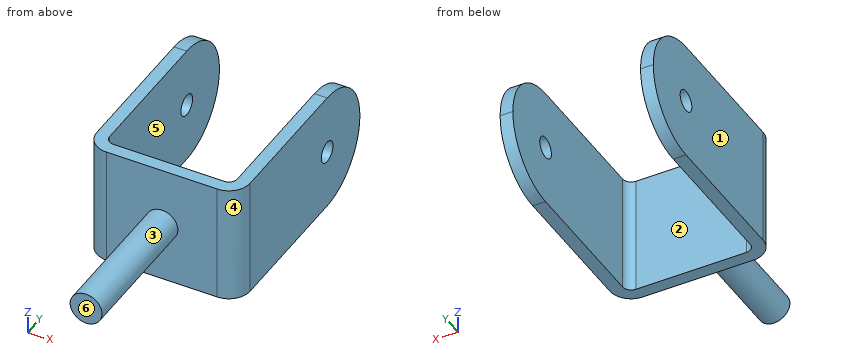
```python
from build123d import *

# Parameters (mm, degrees)
BOSS_EXTRUDE1_DEPTH     = 280
SKETCH2_R               = 25
CUT_EXTRUDE3_DEPTH      = 1
CUT_EXTRUDE3_DEPTH_BACK = 399
SKETCH4_R               = 37.5
BOSS_EXTRUDE2_DEPTH     = 325


with BuildPart() as part:
    # Sketch1 → Boss-Extrude1 (new body)
    with BuildSketch(Plane.XY):
        with BuildLine():
            Line((-130, 0), (130, 0))
            ThreePointArc((130, 0), (165.355339059, 14.644660941), (180, 50))
            Line((180, 50), (180, 520))
            Line((180, 520), (150, 520))
            Line((150, 520), (150, 50))
            ThreePointArc((150, 50), (144.142135624, 35.857864376), (130, 30))
            Line((130, 30), (-130, 30))
            ThreePointArc((-130, 30), (-144.142135624, 35.857864376), (-150, 50))
            Line((-150, 50), (-150, 520))
            Line((-150, 520), (-180, 520))
            Line((-180, 520), (-180, 50))
            ThreePointArc((-180, 50), (-165.355339059, 14.644660941), (-130, 0))
        make_face()
    extrude(amount=BOSS_EXTRUDE1_DEPTH)

    # Sketch2 → Cut-Extrude3 (cut, two sides)
    with BuildSketch(Plane.ZY.offset(180)) as cut_extrude3_sk:
        with BuildLine():
            Line((280, 520), (140, 520))
            ThreePointArc((140, 520), (238.994949366, 478.994949366), (280, 380))
            Line((280, 380), (280, 520))
        make_face()
        with BuildLine():
            Line((0, 520), (0, 380))
            ThreePointArc((0, 380), (41.005050634, 478.994949366), (140, 520))
            Line((140, 520), (0, 520))
        make_face()
        with Locations((140, 380)):
            Circle(SKETCH2_R)
    extrude(amount=CUT_EXTRUDE3_DEPTH, mode=Mode.SUBTRACT)
    extrude(cut_extrude3_sk.sketch, amount=-CUT_EXTRUDE3_DEPTH_BACK, mode=Mode.SUBTRACT)

    # Sketch4 → Boss-Extrude2 (add)
    with BuildSketch(Plane.XZ):
        with Locations((0, 140)):
            Circle(SKETCH4_R)
    extrude(amount=BOSS_EXTRUDE2_DEPTH)


solid = part.part
```
Geometry check sheet. Reference: the model listing, model coordinates, mm. Face numbers are marked on the shaded views. A direction names the side the tool comes from. Give positions to 0.01 mm unless a question says otherwise; leave off trailing zeros. Order: outer loops, then holes, each group sorted by start corner. A loop starts at its lowest first (then second) coordinate and runs counter-clockwise, first axis right, second up.
1. Section check C-C, the plane z = 221. Enter the section's corners in (x, y).
2. Section check B-B, the plane x = 0. Enter the section's corners in (y, z).
3. Access from +Z, -Z, +X, -X, +Y, -Y to the whole of each face (thin tool, end or side, straight path). Record for the marked faces 1, 2 and 3.
4. Thickness scan on L1, parallel to X at y = 440.5, z = 234; L2, parallel to Y at x = -81.5, z = 242.5; L3, parallel to Y at x = 168, z = 140. Record the ranges inside material, lowest first.
5. Section check D-D, the plane y = 452. Enter the section's corners in (x, z).
6. Release check for a two-part mould opening along X. For the marked faces 4, 5 and 6 record: pulls with the +X half, pulls with the -X half, needs draft (parallel to the pull), parting line crosses it, or undercut.
7. Gauge pin test, flat end, axial feed: pin 1 Ø2 at (y, z) = (-116, 124) entering from +X. Record the tip position at first contact, or that the pin passes through.
8. Section check A-A, the plane y = 310.5. Enter the section's corners in (x, z), and give its area (3 significant figures).
Values follow:
1. outline: (-180, 50) arc R50 ccw to (-130, 0) - (130, 0) arc R50 ccw to (180, 50) - (180, 494.19) - (150, 494.19) - (150, 50) arc R20 cw to (130, 30) - (-130, 30) arc R20 cw to (-150, 50) - (-150, 494.19) - (-180, 494.19) - close
2. outline: (-325, 102.5) - (0, 102.5) - (0, 0) - (30, 0) - (30, 280) - (0, 280) - (0, 177.5) - (-325, 177.5) - close
3. face 1: +Z, -Z, -X, +Y, -Y
3. face 2: +Z, -Z, +Y
3. face 3: -Y
4. L1: x = -180 to -150, 150 to 180
4. L2: y = 0 to 30
4. L3: y = 17.5 to 355, 405 to 520
5. outline: (-180, 19.93) - (-150, 19.93) - (-150, 260.07) - (-180, 260.07) - close; (150, 19.93) - (180, 19.93) - (180, 260.07) - (150, 260.07) - close
6. face 4: pulls with the +X half
6. face 5: undercut
6. face 6: needs draft
7. pin 1: stops at x = 34.37
8. outline: (-180, 0) - (-150, 0) - (-150, 280) - (-180, 280) - close; (150, 0) - (180, 0) - (180, 280) - (150, 280) - close
8. area: 16,800 mm2
